Build history of the part. All positions in model axes, mm. A direction names the side the tool comes from. Give positions to 0.01 mm unless a question says otherwise; leave off trailing zeros. Write each loop counter-clockwise with the first axis right and the second up, starting at its lowest first coordinate (ties: lowest second). Pieces come first, ordered by that corner, then holes. Notation, with made-up numbers: (50, 22) -> (82, 22) arc R17 cw to (82, 33) -> close; hole circle Ø2 at (1, -2.5). An arc over 180 degrees is marked (long way). Put each result on its own line as item: value. Start each with the question number.
Item 1: Tool access for faces 5 (the flat face through (154, 203.2, 13)), 6 (the flat face through (0, 165, 13)), 7 (the flat face through (-97, 76.2, 13)): list every direction of +Z, -Z, +X, -X, +Y, -Y with a clear straight run to the whole face (end or side of a thin tool).
Item 2: Slice it at A-A, the plane y = 101.6. List the corners of the cut face in (x, z).
Item 3: Drill centre lines: line 1 along X through (y, z) = (42, 2); line 2 along Y through (x, z) = (-78.5, 3.5); line 3 along X through (y, z) = (90, 22). Where is each one in solid material? Low to high.
Item 4: Slice it at D-D, the plane x = -69.5. List the corners of the cut face in (y, z), plus the area to 3 significant figures.
Item 5: Flat gauge pins, fed straight in: pin 1 Ø12.5 at (x, z) = (-141, 17.5) entering from -Y; pin 2 Ø1.5 at (x, y) = (-121.5, 75) entering from +Z; pin 3 Ø12.5 at (y, z) = (38, 9.5) entering from -X; pin 4 Ø1 at (x, z) = (-37.5, 7.5) entering from +Y. Where does each tip first touch, or does it go through?
Item 6: Slice it at B-B, the plane z = 16.75. List the corners of the cut face in (x, y), plus the area to 3 significant figures.
Item 7: Slice it at C-C, the plane y = 184. List the corners of the cut face in (x, z).
Item 8: Two-plate mould, pull along X, no slides. Class faces 1 (the cylindrical face through (-176.76, 102.16, 12.52)), 2 (the flat face through (-203.2, 101, 13)), 3 (the flat face through (304.8, 100, 13)), 4 (the flat face through (104, 103, 0)): pulls with the +X half, pulls with the -X half, needs draft (parallel to the pull), parting line crosses it, or undercut.
```python
from build123d import *

# Parameters (mm, degrees)
F0_W     = 203.2
F0_H     = 50.8
F0_R     = 12.7
F1_DEPTH = 25.4
F2_R     = 12.7
F3_R     = 12.7


with BuildPart() as f1:
    # F0 (on Top) → F1 (new body)
    with BuildSketch(Plane.XY):
        Polygon((0, 76.2), (0, 0), (304.8, 0), (304.8, 203.2), (0, 203.2), (0, 127), align=None)
        with Locations((-101.6, 101.6)):
            Rectangle(F0_W, F0_H)
        with Locations((-164.072603, 101.6)):
            Circle(F0_R, mode=Mode.SUBTRACT)
    extrude(amount=F1_DEPTH)

    # F2
    f2_edges = [f1.edges().sort_by_distance(p)[0] for p in [
        (0, 127, 12.7),
        (-203.2, 127, 12.7),
        (-203.2, 76.2, 12.7),
    ]]
    fillet(f2_edges, radius=F2_R)

    # F3
    f3_edges = [f1.edges().sort_by_distance(p)[0] for p in [
        (0, 203.2, 12.7),
        (304.8, 203.2, 12.7),
        (304.8, 0, 12.7),
        (0, 0, 12.7),
    ]]
    fillet(f3_edges, radius=F3_R)


solid = f1.part
```
Values follow:
1. face 5: +Z, -Z, +X, -X, +Y
1. face 6: +Z, -Z, -X, +Y
1. face 7: +Z, -Z, -X, -Y
2. outline: (-203.2, 0) -> (-176.77, 0) -> (-176.77, 25.4) -> (-203.2, 25.4) -> close; (-151.37, 0) -> (304.8, 0) -> (304.8, 25.4) -> (-151.37, 25.4) -> close
3. line 1: 0 to 304.8
3. line 2: 76.2 to 127
3. line 3: -203.2 to -169.24, -158.9 to 304.8
4. outline: (76.2, 0) -> (127, 0) -> (127, 25.4) -> (76.2, 25.4) -> close
4. area: 1,290 mm2
5. pin 1: y = 76.2
5. pin 2: through
5. pin 3: x = 0
5. pin 4: y = 127
6. outline: (-203.2, 88.9) arc R12.7 ccw to (-190.5, 76.2) -> (0, 76.2) -> (0, 12.7) arc R12.7 ccw to (12.7, 0) -> (292.1, 0) arc R12.7 ccw to (304.8, 12.7) -> (304.8, 190.5) arc R12.7 ccw to (292.1, 203.2) -> (12.7, 203.2) arc R12.7 ccw to (0, 190.5) -> (0, 139.7) arc R12.7 cw to (-12.7, 127) -> (-190.5, 127) arc R12.7 ccw to (-203.2, 114.3) -> close; hole circle Ø25.4 at (-164.07, 101.6)
6. area: 71,600 mm2
7. outline: (0, 0) -> (304.8, 0) -> (304.8, 25.4) -> (0, 25.4) -> close
8. face 1: undercut
8. face 2: pulls with the -X half
8. face 3: pulls with the +X half
8. face 4: needs draft
